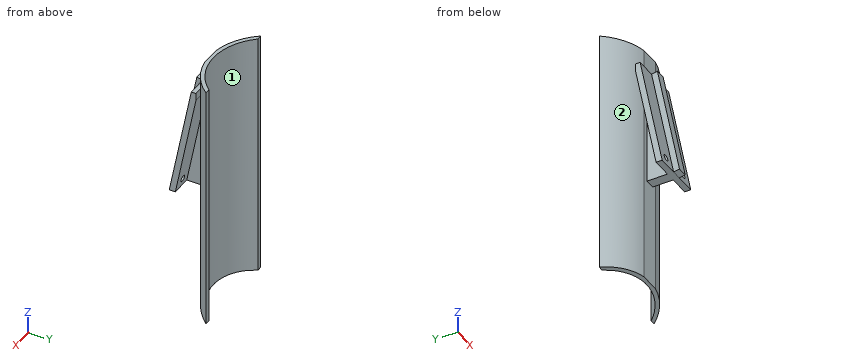
```python
from build123d import *

# Parameters (mm, degrees)
MAIN_DEPTH           = 125
SKETCH2_R            = 25
BEHINDCUT_DEPTH      = 3.605022946
CENTRALSUPPORT_DEPTH = 2.5
SIDESUPPORT_DEPTH    = 12.5
HOLEFIX_REACH        = 37.219
SKETCH6_R            = 1.6
SKETCH9_W            = 5
SKETCH9_H            = 58
BOSS_EXTRUDE4_DEPTH  = 3


with BuildPart() as part:
    # Sketch1 → Main (new body)
    with BuildSketch(Plane.XY):
        with BuildLine():
            Line((-24, 0), (-21.44761059, 0))
            ThreePointArc((-21.44761059, 0), (0, -10), (21.44761059, 0))
            Line((21.44761059, 0), (24, 0))
            ThreePointArc((24, 0), (15.613340762, -7.616861444), (5, -11.580398915))
            Line((5, -11.580398915), (-5, -11.580398915))
            ThreePointArc((-5, -11.580398915), (-15.613340762, -7.616861444), (-24, 0))
        make_face()
    extrude(amount=MAIN_DEPTH)

    # Sketch2 → BehindCut (cut, through all)
    with BuildSketch(Plane(origin=(0, 0, 0), x_dir=(1, 0, 0), z_dir=(0, 0.224951054, 0.974370065))):
        Circle(SKETCH2_R)
    extrude(amount=-BEHINDCUT_DEPTH, mode=Mode.SUBTRACT)

    # Sketch4 → CentralSupport (add, symmetric)
    with BuildSketch(Plane(origin=(0, 0, 0), x_dir=(0, 0, -1), z_dir=(1, 0, 0))):
        Polygon((-113, -11.580398915), (-56.06562336, -11.580398915), (-56.06562336, -24.979884357), (-113, -13.912962625), align=None)
    extrude(amount=CENTRALSUPPORT_DEPTH, both=True)

    # Sketch5 → SideSupport (add, symmetric)
    with BuildSketch(Plane(origin=(0, 0, 0), x_dir=(0, 0, -1), z_dir=(1, 0, 0))):
        Polygon((-56.06562336, -24.979884357), (-113, -13.912962625), (-113, -11.580398915), (-109.277470807, -11.580398915), (-56.06562336, -21.923734272), align=None)
    extrude(amount=SIDESUPPORT_DEPTH, both=True)

    # Sketch6 → HoleFix (cut, up to next)
    with BuildSketch(Plane(origin=(0, -34.571690998, 6.720055984), x_dir=(-1, 0, 0), z_dir=(0, -0.981627183, 0.190808995)), mode=Mode.PRIVATE) as holefix_sk1:
        with Locations((7.5, -55.269153308)):
            Circle(SKETCH6_R)
    holefix_tool1 = extrude(holefix_sk1.sketch, amount=-HOLEFIX_REACH, mode=Mode.PRIVATE) & part.part
    add(holefix_tool1.solids().sort_by_distance((-7.5, -24.025839, 60.973759))[0], mode=Mode.SUBTRACT)
    # Sketch6 → HoleFix (cut, up to next)
    with BuildSketch(Plane(origin=(0, -34.571690998, 6.720055984), x_dir=(-1, 0, 0), z_dir=(0, -0.981627183, 0.190808995)), mode=Mode.PRIVATE) as holefix_sk2:
        with Locations((-7.5, -55.269153308)):
            Circle(SKETCH6_R)
    holefix_tool2 = extrude(holefix_sk2.sketch, amount=-HOLEFIX_REACH, mode=Mode.PRIVATE) & part.part
    add(holefix_tool2.solids().sort_by_distance((7.5, -24.025839, 60.973759))[0], mode=Mode.SUBTRACT)

    # Sketch9 → Boss-Extrude4 (add)
    with BuildSketch(Plane(origin=(0, -34.571690998, 6.720055984), x_dir=(-1, 0, 0), z_dir=(0, -0.981627183, 0.190808995))):
        with Locations((0, -79.269153308)):
            Rectangle(SKETCH9_W, SKETCH9_H)
    extrude(amount=BOSS_EXTRUDE4_DEPTH)


solid = part.part
```
Part model, mm, in its own coordinate system. Face numbers are marked on the shaded views. Give positions to 0.01 mm unless a question says otherwise; leave off trailing zeros. Order: outer loops, then holes, each group sorted by start corner. A loop starts at its lowest first (then second) coordinate and runs counter-clockwise, first axis right, second up. Notation, with made-up numbers: M -19,88.5 L -6,88.5 A13 cw -6,110.5 Z; hole C 83.25,14 d2. An arc over 180 degrees is marked long. Use a Markdown table: item, result. Add a question column.
(1) Mould opens along Y. For the marked faces 1 and 2 say: +Y half, -Y half, draft (parallel to the pull), parting line (faces both ways), or undercut.
(2) Drop flat-ended pins along their axis: P1, Ø10, axis at x = -11, z = 79.5, coming from the -Y side; P2, Ø14.5, axis at y = -15.5, z = 93.5, coming from the +X side; P3, Ø4, axis at y = -19.5, z = 76, coming from the -X side; P4, Ø1, axis at y = -17, z = 55.5, coming from the +X side. Give the stop position or say it passes through.
(3) Saw through at A-A, the plane x = -7. Give the cut face in (y, z), and give its area (3 significant figures).
(4) Saw through at C-C, the plane y = -7. Give the cut face in (x, z), and give its area (3 significant figures).
(5) Saw through at B-B, the plane z = 47.5. Give the cut face in (x, y).
(6) Saw through at D-D, the plane x = 0. Give the cut face in (y, z), and give its area (3 significant figures).
(7) Probe line 1 along X through (y, z) = (-7, 50.5); line 2 along X through (y, z) = (-0.75, 84); line 3 along X through (y, z) = (-14, 76). List the from-to ranges inside material, lowest first. Write a range as [from, to].
Answer key:
| question | item | result |
|---|---|---|
| 1 | face 1 | +Y half |
| 1 | face 2 | undercut |
| 2 | P1 | y = -21.4 |
| 2 | P2 | x = 14.52 |
| 2 | P3 | x = -12.5 |
| 2 | P4 | through |
| 3 | outline | M -24.98,56.07 L -21.92,56.07 L -21.37,58.91 L -24.32,59.48 Z; M -23.74,62.47 L -20.79,61.89 L -11.58,109.28 L -11.58,113 L -13.91,113 Z; M -11.17,2.58 L -9.11,2.1 L -9.11,125 L -11.17,125 Z |
| 3 | area | 416 mm^2 |
| 4 | outline | M -16.58,1.62 L -12.61,1.62 L -12.61,125 L -16.58,125 Z; M 12.61,1.62 L 16.58,1.62 L 16.58,125 L 12.61,125 Z |
| 4 | area | 981 mm^2 |
| 5 | outline | M -24,0 A30 ccw -5,-11.58 L 5,-11.58 A30 ccw 24,0 L 21.45,0 A28 cw -21.45,0 Z |
| 6 | outline | M -27.92,56.64 L -24.98,56.07 L -11.58,56.07 L -11.58,2.67 L -10,2.31 L -10,125 L -11.58,125 L -11.58,113 L -13.91,113 L -16.86,113.57 Z |
| 6 | area | 815 mm^2 |
| 7 | line 1 | [-16.58, -12.61], [12.61, 16.58] |
| 7 | line 2 | [-23.42, -20.8], [20.8, 23.42] |
| 7 | line 3 | [-2.5, 2.5] |
